Geometry: see drawing. Coordinates: mm, zero at the bounding-box minimum. Coordinates: 2 decimals unless noted, no trailing zeros. Loops run counter-clockwise (first coordinate to the right, second up) from the corner with the lowest first, then second, coordinate; pieces in that order, holes last. Notation, with made-up numbers: (27, 34) -> (57, 34) arc R30 cw to (57, 71) -> close; hole circle Ø3 at (24.5, 77). An arc over 180 degrees is marked (long way). One line per question, with ' | ' between items. Start each with the question number.
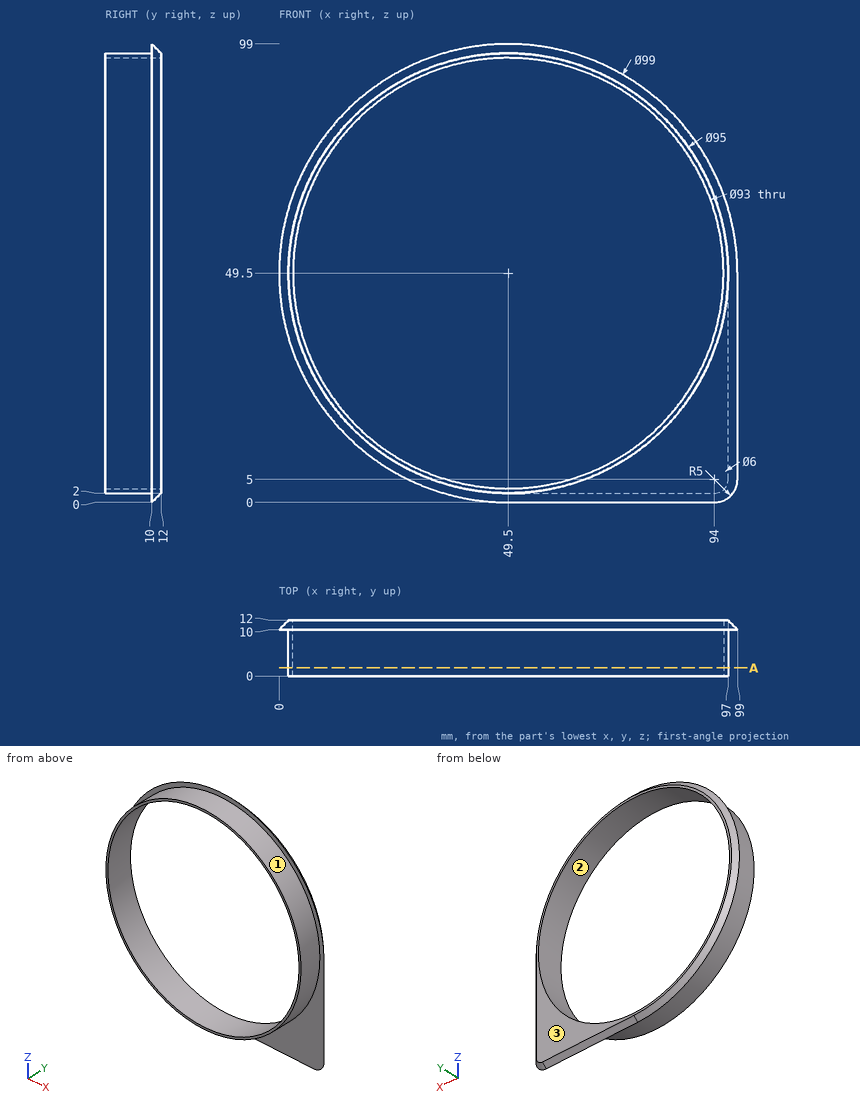
(1) Ray query, L1, parallel to Z at x = 49.5, y = 7.5; L2, parallel to Z at x = 86, y = 11; L3, parallel to X at y = 1.5, z = 15. Return the intervals inside material, ascending.
(2) Draft query along Z for the marked faces 1, 2 and 3. Return one class per face: pulls with the +Z half, pulls with the -Z half, needs draft (parallel to the pull), parting line crosses it, or undercut.
(3) Contact query for flat-ended pins moving along their axis: pin 1 Ø4 at (x, y) = (60, 3.5) entering from -Z; pin 2 Ø5 at (x, z) = (21, 86) entering from +Y; pin 3 Ø2 at (y, z) = (4, 13) entering from -X. Output: stop coordinate, or through.
(4) Cut plane A-A, the plane y = 1.75. Return the cut outline in (x, z).
Here are the results:
1) L1: z = 2 to 3, 96 to 97 | L2: z = 1 to 20.69, 78.31 to 81.44 | L3: x = 16.85 to 18.32, 80.68 to 82.15
2) face 1: parting line crosses it | face 2: undercut | face 3: needs draft
3) pin 1: stops at z = 2.77 | pin 2: stops at y = 12 | pin 3: stops at x = 17.94
4) outline: circle Ø95 at (49.5, 49.5); hole circle Ø93 at (49.5, 49.5)
